Input: dimensioned drawing with shaded views. Units: mm. Origin: part minimum x, y, z. A direction names the side the tool comes from. Coordinates: 2 decimals unless noted, no trailing zeros. Order: outer loops, then holes, each group sorted by start corner. A loop starts at its lowest first (then second) coordinate and runs counter-clockwise, first axis right, second up.
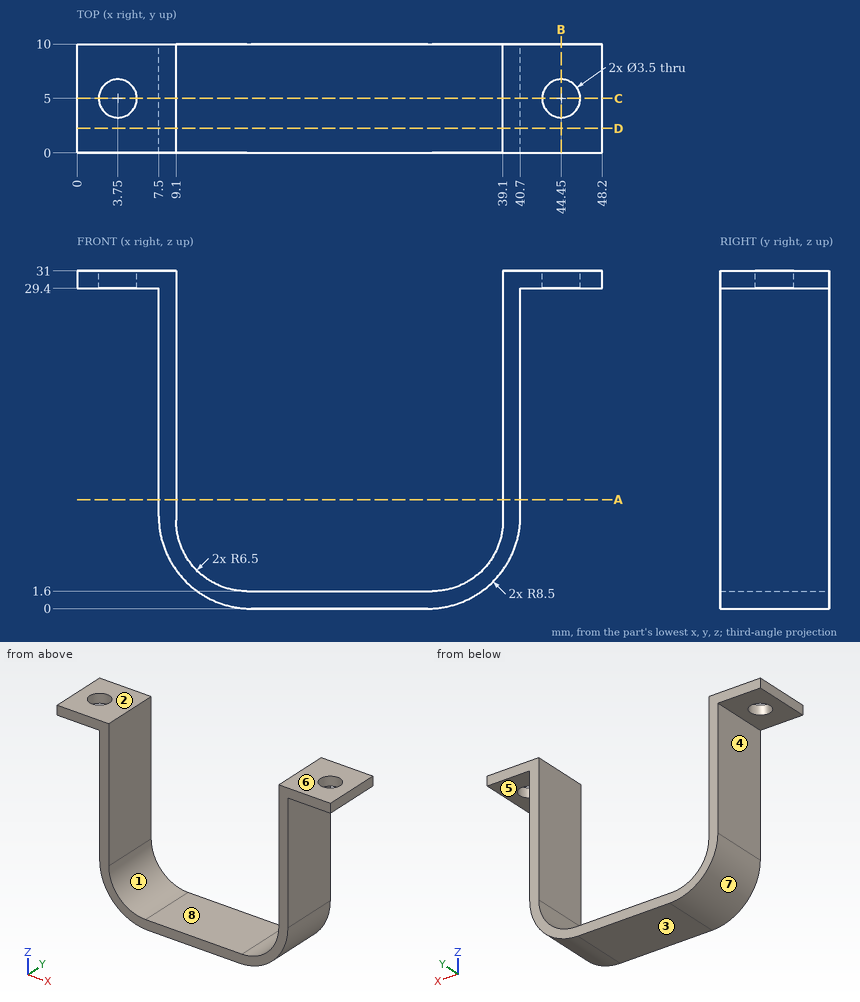
1. Section query D-D on y = 2.25. Return loops of the section in (x, z), plus the area to 3 significant figures.
Findings:
outline: (0, 29.4) - (7.5, 29.4) - (7.5, 8.5) arc R8.5 ccw to (16, 0) - (32.2, 0) arc R8.5 ccw to (40.7, 8.5) - (40.7, 29.4) - (48.2, 29.4) - (48.2, 31) - (39.1, 31) - (39.1, 8.1) arc R6.5 cw to (32.6, 1.6) - (15.6, 1.6) arc R6.5 cw to (9.1, 8.1) - (9.1, 31) - (0, 31) - close
area: 158 mm2
2. Ray query, line 1 (X direction, y = 5, z = 29.95); line 2 (X direction, y = 0.5, z = 18); line 3 (Y direction, x = 3.75, z = 30.15). Return the intervals inside material, ascending.
Findings:
line 1: x = 0 to 2, 5.5 to 9.1, 39.1 to 42.7, 46.2 to 48.2
line 2: x = 7.5 to 9.1, 39.1 to 40.7
line 3: y = 0 to 3.25, 6.75 to 10
3. Pin query (flat end, axial travel): P1, Ø5, axis at y = 5, z = 17.5, coming from the -X side; P2, Ø1.5, axis at x = 36.5, z = 14, coming from the +Y side; P3, Ø2, axis at y = 6, z = 20.5, coming from the +X side; P4, Ø5.5, axis at x = 3.75, y = 5, coming from the -Z side. Return the tip coordinate at first contact, or that it passes through.
Findings:
P1: stops at x = 7.5
P2: passes through
P3: stops at x = 40.7
P4: stops at z = 29.4
4. Draft query along X for the marked faces 6, 7 and 8. Return one class per face: released by +X, released by -X, zero draft, split by the parting line, or undercut.
Findings:
face 6: zero draft
face 7: released by -X
face 8: undercut
5. Section query C-C on y = 5. Return loops of the section in (x, z), plus the area to 3 significant figures.
Findings:
outline: (0, 29.4) - (2, 29.4) - (2, 31) - (0, 31) - close; (5.5, 29.4) - (7.5, 29.4) - (7.5, 8.5) arc R8.5 ccw to (16, 0) - (32.2, 0) arc R8.5 ccw to (40.7, 8.5) - (40.7, 29.4) - (42.7, 29.4) - (42.7, 31) - (39.1, 31) - (39.1, 8.1) arc R6.5 cw to (32.6, 1.6) - (15.6, 1.6) arc R6.5 cw to (9.1, 8.1) - (9.1, 31) - (5.5, 31) - close; (46.2, 29.4) - (48.2, 29.4) - (48.2, 31) - (46.2, 31) - close
area: 147 mm2
6. Section query B-B on x = 44.45. Return loops of the section in (y, z).
Findings:
outline: (0, 29.4) - (3.25, 29.4) - (3.25, 31) - (0, 31) - close; (6.75, 29.4) - (10, 29.4) - (10, 31) - (6.75, 31) - close
7. Section query A-A on z = 10. Return loops of the section in (x, y).
Findings:
outline: (7.5, 0) - (9.1, 0) - (9.1, 10) - (7.5, 10) - close; (39.1, 0) - (40.7, 0) - (40.7, 10) - (39.1, 10) - close
8. Access query for the marked faces 1, 2, 3, 4 and 5. Directions: +Z, -Z, +X, -X, +Y, -Y. A direction counts if a zero-diameter tool reaches every point of the face in a straight line with its end or side. Return the directions, or none.
Findings:
face 1: +Z, +Y, -Y
face 2: +Z, +X, -X, +Y, -Y
face 3: -Z, +X, -X, +Y, -Y
face 4: -Z, -X, +Y, -Y
face 5: -Z, +X, +Y, -Y
